Build history of the part. All positions in model axes, mm. Round coordinates to 2 decimals unless told otherwise and drop trailing zeros. Loops run counter-clockwise (first coordinate to the right, second up) from the corner with the lowest first, then second, coordinate; pieces in that order, holes last. Notation, with made-up numbers: (37.25, -23) - (51.25, -23) arc R11 ccw to (51.25, -17) - close; hole circle Ø7 at (60.5, -2). An arc over 180 degrees is marked (long way). Use a Markdown table: item, result.
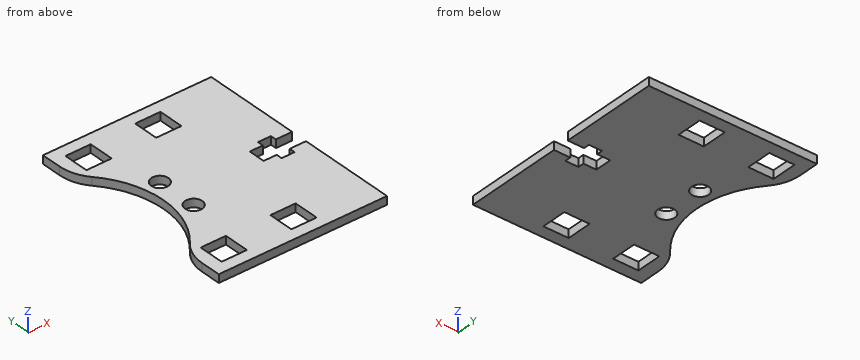
from build123d import *

# Parameters (mm, degrees)
SKETCH_1_R      = 2.1
SKETCH_1_W      = 6.2
SKETCH_1_H      = 6.2
EXTRUDE_1_DEPTH = 2
FILLET_1_R      = 10


with BuildPart() as part:
    # 草图1 → 凸台-拉伸1 (new body)
    with BuildSketch(Plane.XY):
        with BuildLine():
            Line((64.766222961, -26), (23.516222961, -26))
            Line((23.516222961, -26), (23.516222961, -16.9))
            ThreePointArc((23.516222961, -16.9), (31.401260639, 0), (23.516222961, 16.9))
            Line((23.516222961, 16.9), (23.516222961, 26))
            Line((23.516222961, 26), (64.766222961, 26))
            Line((64.766222961, 26), (64.766222961, 2.05))
            Line((64.766222961, 2.05), (60.766222961, 2.05))
            Line((60.766222961, 2.05), (60.766222961, 3.5))
            Line((60.766222961, 3.5), (57.566222961, 3.5))
            Line((57.566222961, 3.5), (57.566222961, 2.05))
            Line((57.566222961, 2.05), (54.366222961, 2.05))
            Line((54.366222961, 2.05), (54.366222961, -2.05))
            Line((54.366222961, -2.05), (57.566222961, -2.05))
            Line((57.566222961, -2.05), (57.566222961, -3.5))
            Line((57.566222961, -3.5), (60.766222961, -3.5))
            Line((60.766222961, -3.5), (60.766222961, -2.05))
            Line((60.766222961, -2.05), (64.766222961, -2.05))
            Line((64.766222961, -2.05), (64.766222961, -26))
        make_face()
        with Locations((34.766222961, 5)):
            Circle(SKETCH_1_R, mode=Mode.SUBTRACT)
        with Locations(Location((34.766222961, -5, 0), (0, 0, 180))):
            Circle(SKETCH_1_R, mode=Mode.SUBTRACT)
        with Locations((46.816222961, -20)):
            Rectangle(SKETCH_1_W, SKETCH_1_H, mode=Mode.SUBTRACT)
        with Locations((29.716222961, -20)):
            Rectangle(SKETCH_1_W, SKETCH_1_H, mode=Mode.SUBTRACT)
        with Locations((29.716222961, 20)):
            Rectangle(SKETCH_1_W, SKETCH_1_H, mode=Mode.SUBTRACT)
        with Locations((46.816222961, 20)):
            Rectangle(SKETCH_1_W, SKETCH_1_H, mode=Mode.SUBTRACT)
    extrude(amount=EXTRUDE_1_DEPTH)

    # 圆角1
    fillet_1_edges = [part.edges().sort_by_distance(p)[0] for p in [
        (23.516222961, -16.9, 1),
        (23.516222961, 16.9, 1),
    ]]
    fillet(fillet_1_edges, radius=FILLET_1_R)


solid = part.part
Q1. Cut at A-A, the plane x = 44.5. List the corners of the cut face in (y, z), plus the area to 3 significant figures.
Results found:
| item | result |
|---|---|
| outline | (-26, 0) - (-23.1, 0) - (-23.1, 2) - (-26, 2) - close; (-16.9, 0) - (16.9, 0) - (16.9, 2) - (-16.9, 2) - close; (23.1, 0) - (26, 0) - (26, 2) - (23.1, 2) - close |
| area | 79.2 mm2 |
Q2. Probe line 1 (Y direction, x = 48, z = 0.65); line 2 (Y direction, x = 35.5, z = 1.2); line 3 (Y direction, x = 63, z = 0.7). List the from-to ranges inside material, lowest first.
Results found:
| item | result |
|---|---|
| line 1 | y = -26 to -23.1, -16.9 to 16.9, 23.1 to 26 |
| line 2 | y = -26 to -6.97, -3.03 to 3.03, 6.97 to 26 |
| line 3 | y = -26 to -2.05, 2.05 to 26 |
Q3. Cut at D-D, the plane z = 0.4. Count the separate pieces of the cut face and the enclosed holes in it, plus the area to 3 significant figures.
Results found:
| item | result |
|---|---|
| separate pieces | 1 |
| enclosed holes | 6 |
| area | 1,720 mm2 |
Q4. Cut at C-C, the plane y = -5. List the corners of the cut face in (x, z).
Results found:
| item | result |
|---|---|
| outline | (30.83, 0) - (32.67, 0) - (32.67, 2) - (30.83, 2) - close; (36.87, 0) - (64.77, 0) - (64.77, 2) - (36.87, 2) - close |
Q5. Cut at B-B, the plane y = 22.5. List the corners of the cut face in (x, z), plus the area to 3 significant figures.
Results found:
| item | result |
|---|---|
| outline | (23.52, 0) - (26.62, 0) - (26.62, 2) - (23.52, 2) - close; (32.82, 0) - (43.72, 0) - (43.72, 2) - (32.82, 2) - close; (49.92, 0) - (64.77, 0) - (64.77, 2) - (49.92, 2) - close |
| area | 57.7 mm2 |
Q6. Drop flat-ended pins along their axis: pin 1 (0.7 mm diameter, centred on y = -2.5, z = 1, fed in from -X); pin 2 (1.2 mm diameter, centred on y = 3, z = 0.5, fed in from -X). Give the stop position or say it passes through.
Results found:
| item | result |
|---|---|
| pin 1 | stops at x = 31.22 |
| pin 2 | stops at x = 31.11 |
